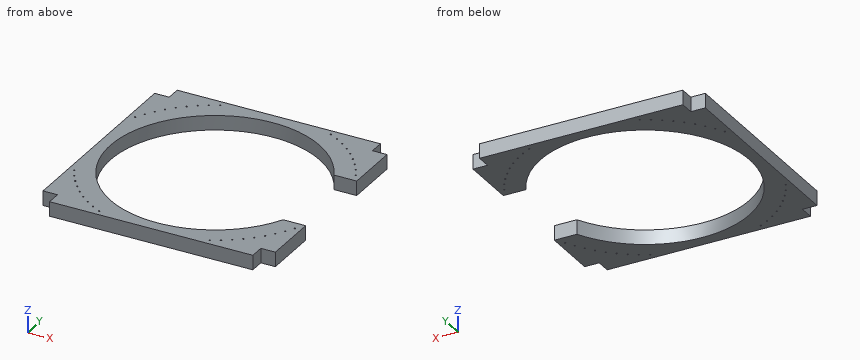
from build123d import *

# Parameters (mm, degrees)
ESQUISSE1_R        = 0.25
BOSS_EXTRU_1_DEPTH = 5
ESQUISSE2_W        = 5
ESQUISSE2_H        = 5
CR_NEAUX_DEPTH     = 5


with BuildPart() as part:
    # Esquisse1 → Boss.-Extru.1 (new body)
    with BuildSketch(Plane.XY):
        with BuildLine():
            Line((0, 80), (80, 80))
            Line((80, 80), (80, 56))
            Line((80, 56), (72.249030993, 56))
            ThreePointArc((72.249030993, 56), (4, 40), (72.249030993, 24))
            Line((72.249030993, 24), (80, 24))
            Line((80, 24), (80, 0))
            Line((80, 0), (0, 0))
            Line((0, 0), (0, 80))
        make_face()
        with Locations((2.018546053, 59.069849399)):
            Circle(ESQUISSE1_R, mode=Mode.SUBTRACT)
        with Locations((7.641889366, 67.553632723)):
            Circle(ESQUISSE1_R, mode=Mode.SUBTRACT)
        with Locations((9.9479618, 70.0520382)):
            Circle(ESQUISSE1_R, mode=Mode.SUBTRACT)
        with Locations((3.664453699, 62.04491041)):
            Circle(ESQUISSE1_R, mode=Mode.SUBTRACT)
        with Locations((5.542908841, 64.878883995)):
            Circle(ESQUISSE1_R, mode=Mode.SUBTRACT)
        with Locations(Location((20.930150601, 77.981453947, 0), (0, 0, 180))):
            Circle(ESQUISSE1_R, mode=Mode.SUBTRACT)
        with Locations(Location((17.95508959, 76.335546301, 0), (0, 0, 180))):
            Circle(ESQUISSE1_R, mode=Mode.SUBTRACT)
        with Locations(Location((15.121116005, 74.457091159, 0), (0, 0, 180))):
            Circle(ESQUISSE1_R, mode=Mode.SUBTRACT)
        with Locations(Location((12.446367277, 72.358110634, 0), (0, 0, 180))):
            Circle(ESQUISSE1_R, mode=Mode.SUBTRACT)
        with Locations((67.553632723, 72.358110634)):
            Circle(ESQUISSE1_R, mode=Mode.SUBTRACT)
        with Locations((64.878883995, 74.457091159)):
            Circle(ESQUISSE1_R, mode=Mode.SUBTRACT)
        with Locations((62.04491041, 76.335546301)):
            Circle(ESQUISSE1_R, mode=Mode.SUBTRACT)
        with Locations((59.069849399, 77.981453947)):
            Circle(ESQUISSE1_R, mode=Mode.SUBTRACT)
        with Locations(Location((74.457091159, 64.878883995, 0), (0, 0, 180))):
            Circle(ESQUISSE1_R, mode=Mode.SUBTRACT)
        with Locations(Location((76.335546301, 62.04491041, 0), (0, 0, 180))):
            Circle(ESQUISSE1_R, mode=Mode.SUBTRACT)
        with Locations(Location((70.0520382, 70.0520382, 0), (0, 0, 180))):
            Circle(ESQUISSE1_R, mode=Mode.SUBTRACT)
        with Locations(Location((72.358110634, 67.553632723, 0), (0, 0, 180))):
            Circle(ESQUISSE1_R, mode=Mode.SUBTRACT)
        with Locations(Location((77.981453947, 59.069849399, 0), (0, 0, 180))):
            Circle(ESQUISSE1_R, mode=Mode.SUBTRACT)
        with Locations((77.981453947, 20.930150601)):
            Circle(ESQUISSE1_R, mode=Mode.SUBTRACT)
        with Locations((72.358110634, 12.446367277)):
            Circle(ESQUISSE1_R, mode=Mode.SUBTRACT)
        with Locations((70.0520382, 9.9479618)):
            Circle(ESQUISSE1_R, mode=Mode.SUBTRACT)
        with Locations((76.335546301, 17.95508959)):
            Circle(ESQUISSE1_R, mode=Mode.SUBTRACT)
        with Locations((74.457091159, 15.121116005)):
            Circle(ESQUISSE1_R, mode=Mode.SUBTRACT)
        with Locations(Location((59.069849399, 2.018546053, 0), (0, 0, 180))):
            Circle(ESQUISSE1_R, mode=Mode.SUBTRACT)
        with Locations(Location((62.04491041, 3.664453699, 0), (0, 0, 180))):
            Circle(ESQUISSE1_R, mode=Mode.SUBTRACT)
        with Locations(Location((64.878883995, 5.542908841, 0), (0, 0, 180))):
            Circle(ESQUISSE1_R, mode=Mode.SUBTRACT)
        with Locations(Location((67.553632723, 7.641889366, 0), (0, 0, 180))):
            Circle(ESQUISSE1_R, mode=Mode.SUBTRACT)
        with Locations((12.446367277, 7.641889366)):
            Circle(ESQUISSE1_R, mode=Mode.SUBTRACT)
        with Locations((15.121116005, 5.542908841)):
            Circle(ESQUISSE1_R, mode=Mode.SUBTRACT)
        with Locations((17.95508959, 3.664453699)):
            Circle(ESQUISSE1_R, mode=Mode.SUBTRACT)
        with Locations((20.930150601, 2.018546053)):
            Circle(ESQUISSE1_R, mode=Mode.SUBTRACT)
        with Locations(Location((5.542908841, 15.121116005, 0), (0, 0, 180))):
            Circle(ESQUISSE1_R, mode=Mode.SUBTRACT)
        with Locations(Location((3.664453699, 17.95508959, 0), (0, 0, 180))):
            Circle(ESQUISSE1_R, mode=Mode.SUBTRACT)
        with Locations(Location((9.9479618, 9.9479618, 0), (0, 0, 180))):
            Circle(ESQUISSE1_R, mode=Mode.SUBTRACT)
        with Locations(Location((7.641889366, 12.446367277, 0), (0, 0, 180))):
            Circle(ESQUISSE1_R, mode=Mode.SUBTRACT)
        with Locations(Location((2.018546053, 20.930150601, 0), (0, 0, 180))):
            Circle(ESQUISSE1_R, mode=Mode.SUBTRACT)
    extrude(amount=BOSS_EXTRU_1_DEPTH)

    # Esquisse2 → Créneaux - (cut)
    with BuildSketch(Plane(origin=(0, 0, 0), x_dir=(-1, 0, 0), z_dir=(0, 0, -1))):
        with Locations((-2.5, 2.5)):
            Rectangle(ESQUISSE2_W, ESQUISSE2_H)
        with Locations((-77.5, 2.5)):
            Rectangle(ESQUISSE2_W, ESQUISSE2_H)
        with Locations((-77.5, 77.5)):
            Rectangle(ESQUISSE2_W, ESQUISSE2_H)
        with Locations((-2.5, 77.5)):
            Rectangle(ESQUISSE2_W, ESQUISSE2_H)
    extrude(amount=-CR_NEAUX_DEPTH, mode=Mode.SUBTRACT)


solid = part.part
Design review of the part built by this model. Coordinates are the model's own, in mm. Give positions to 0.01 mm unless a question says otherwise; leave off trailing zeros. Order: outer loops, then holes, each group sorted by start corner. A loop starts at its lowest first (then second) coordinate and runs counter-clockwise, first axis right, second up.
1. Add section A-A, the plane x = 40. State the section outline as (y, z) points.
Solution:
outline: (0, 0) - (4, 0) - (4, 5) - (0, 5) - close; (76, 0) - (80, 0) - (80, 5) - (76, 5) - close
2. Add section D-D, the plane z = 3.6. State how many separate pieces and enclosed holes the cut face has, then the cut area to 3 significant figures.
Solution:
separate pieces: 1
enclosed holes: 36
area: 2,050 mm2
3. Add section C-C, the plane y = 40. State the section outline as (x, z) points, then the cut area to 3 significant figures.
Solution:
outline: (0, 0) - (4, 0) - (4, 5) - (0, 5) - close
area: 20.0 mm2
4. To check wall thickness, follow L1, parallel to Y at x = 77.5, z = 1.6; L2, parallel to X at y = 15, z = 3.6; L3, parallel to X at y = 18, z = 3.45. State the ranges of each line that lie inside material, in increasing order.
Solution:
L1: y = 5 to 24, 56 to 75
L2: x = 0 to 5.32, 5.76 to 14.1, 65.9 to 74.24, 74.68 to 80
L3: x = 0 to 3.42, 3.91 to 11.5, 68.5 to 76.09, 76.58 to 80
5. For pin 1 Ø2.5 at (x, z) = (77.5, 1.5) entering from +Y; pin 2 Ø2.5 at (x, z) = (78.5, 2.5) entering from -Y; pin 3 Ø2 at (y, z) = (25, 4) entering from -X; pin 4 Ø1.5 at (y, z) = (2.5, 2.5) entering from -X, all flat-tipped, find the tip position at first contact; note any pin that passes through.
Solution:
pin 1: stops at y = 75
pin 2: stops at y = 5
pin 3: stops at x = 0
pin 4: stops at x = 5
6. Add section B-B, the plane x = 23. State the section outline as (y, z) points, then the cut area to 3 significant figures.
Solution:
outline: (0, 0) - (8.27, 0) - (8.27, 5) - (0, 5) - close; (71.73, 0) - (80, 0) - (80, 5) - (71.73, 5) - close
area: 82.7 mm2
